Geometry check sheet. Reference: the model listing, model coordinates, mm. A direction names the side the tool comes from. Coordinates: 2 decimals unless noted, no trailing zeros. Write each loop counter-clockwise with the first axis right and the second up, starting at its lowest first coordinate (ties: lowest second). Pieces come first, ordered by that corner, then holes. Notation, with made-up numbers: (19.25, 46.25) -> (47.25, 46.25) arc R5 ccw to (47.25, 54.25) -> close; hole circle Ø7 at (48, -31.75). An arc over 180 degrees is marked (long way). Answer in a Markdown table with one row per item. Add a question column.
Q1. Release check for a two-part mould opening along Z. For faces 1 (the face through (43.909, 4.829, -77.465)), 2 (the face through (-1, 3.683, -1)), 3 (the face through (-45.4, 9.525, -0.4)) record: pulls with the +Z half, pulls with the -Z half, needs draft (parallel to the pull), parting line crosses it, or undercut.
Q2. Gauge pin test, flat ends, axial feed: P1, Ø3, axis at x = -19.5, z = -28, coming from the +Y side; P2, Ø1.4, axis at x = -19.05, y = 1.778, coming from the -Z side; P3, Ø1.8, axis at x = 19.05, y = 1.778, coming from the -Z side. Record the tip position at first contact, or that the pin passes through.
Q3. Thickness scan on line 1 (Y direction, x = -19.05, z = -75.5); line 2 (Z direction, x = 36, y = 4.25) (3 decimals); line 3 (X direction, y = 3.75, z = -24). Record the ranges inside material, lowest first.
Q4. Section check B-B, the plane x = -7. Record the boundary of the cut face in (y, z) (3 decimals), and give its area (3 significant figures).
Q5. Tool access check on faces 4 (the face through (-43.909, 4.829, -77.465)), 5 (the face through (-27.94, 7, -72)), 6 (the face through (-32.447, 7.741, 65.264)). Record the directions out of +Z, -Z, +X, -X, +Y, -Y that give a thin tool (end or side, any length) a straight path to the whole face; none if there is none.
Q6. Section check A-A, the plane z = 62.5. Record the boundary of the cut face in (x, y) (3 decimals), and give its area (3 significant figures).
```python
from build123d import *

# Parameters (mm, degrees)
SKETCH1_W                      = 91.44
SKETCH1_H                      = 158.75
BOSS_EXTRUDE1_DEPTH            = 9.525
FILLET1_R                      = 6.35
SKETCH2_W                      = 86.36
SKETCH2_H                      = 128.524
CUT_EXTRUDE1_DEPTH             = 5.842
F_4_40_TAPPED_HOLE1_AT_2_COUNT = 2
F_4_40_TAPPED_HOLE1_AT_2_PITCH = 38.1
SKETCH7_R                      = 3.175
CUT_EXTRUDE2_DEPTH             = 5.842
CHAMFER1_SIZE                  = 2.032
CHAMFER1_SIZE2                 = 3.519527241
CUT_EXTRUDE3_REACH             = 94.095
SKETCH8_W                      = 55.88
SKETCH8_H                      = 158.75


with BuildPart() as part:
    # Sketch1 → Boss-Extrude1 (new body)
    with BuildSketch(Plane(origin=(0, 0, 0), x_dir=(1, 0, 0), z_dir=(0, 1, 0))):
        Rectangle(SKETCH1_W, SKETCH1_H)
    extrude(amount=BOSS_EXTRUDE1_DEPTH)

    # Fillet1
    fillet1_edges = [part.edges().sort_by_distance(p)[0] for p in [
        (45.72, 4.7625, 79.375),
        (-45.72, 4.7625, 79.375),
        (-45.72, 4.7625, -79.375),
        (45.72, 4.7625, -79.375),
    ]]
    fillet(fillet1_edges, radius=FILLET1_R)

    # Sketch2 → Cut-Extrude1 (cut)
    with BuildSketch(Plane(origin=(0, 9.525, 0), x_dir=(1, 0, 0), z_dir=(0, 1, 0))):
        Rectangle(SKETCH2_W, SKETCH2_H)
    extrude(amount=-CUT_EXTRUDE1_DEPTH, mode=Mode.SUBTRACT)

    # Sketch5 → #4-40 Tapped Hole1 (revolve, cut)
    with BuildSketch(Plane(origin=(-19.05, 1.778, 79.375), x_dir=(0, -1, 0), z_dir=(1, 0, 0))):
        Polygon((0, 0), (0, 8.273752758), (1.1303, 7.5946), (1.1303, 0), align=None)
    f_4_40_tapped_hole1 = revolve(axis=Axis((-19.05, 1.778, 85.725), (0, 0, -1)), mode=Mode.SUBTRACT)

    # #4-40 Tapped Hole1 at 2: #4-40 Tapped Hole1 ×2
    with Locations(*[(i * F_4_40_TAPPED_HOLE1_AT_2_PITCH, 0, 0) for i in range(1, F_4_40_TAPPED_HOLE1_AT_2_COUNT)]):
        add(f_4_40_tapped_hole1, mode=Mode.SUBTRACT)

    # Sketch7 → Cut-Extrude2 (cut)
    with BuildSketch(Plane(origin=(0, 9.525, 0), x_dir=(1, 0, 0), z_dir=(0, 1, 0))):
        with Locations((-40.005, 64.262)):
            Circle(SKETCH7_R)
        with Locations((40.005, 64.262)):
            Circle(SKETCH7_R)
        with Locations((-40.005, -64.262)):
            Circle(SKETCH7_R)
        with Locations((40.005, -64.262)):
            Circle(SKETCH7_R)
    extrude(amount=-CUT_EXTRUDE2_DEPTH, mode=Mode.SUBTRACT)

    # Mirror1: #4-40 Tapped Hole1 across plane
    add(f_4_40_tapped_hole1.mirror(Plane.XY), mode=Mode.SUBTRACT)

    # Mirror1 copy 1 sketch → Mirror1 copy 1 (revolve, cut)
    with BuildSketch(Plane(origin=(19.05, 1.778, -79.375), x_dir=(0, -1, 0), z_dir=(1, 0, 0))):
        Polygon((0, 0), (0, -8.273752758), (1.1303, -7.5946), (1.1303, 0), align=None)
    revolve(axis=Axis((19.05, 1.778, -85.725), (0, 0, -1)), mode=Mode.SUBTRACT)

    # Chamfer1
    chamfer1_edges = [part.edges().sort_by_distance(p)[0] for p in [
        (43.18, 9.525, 0),
        (-43.18, 9.525, 0),
        (0, 9.525, -64.262),
        (0, 9.525, 64.262),
        (40.005, 9.525, -67.437),
        (-40.005, 9.525, 67.437),
        (40.005, 9.525, 67.437),
        (-40.005, 9.525, -67.437),
    ]]
    chamfer1_side = [part.faces().sort_by_distance(p)[0] for p in [
        (0, 9.525, -77.542983731),
    ]]
    chamfer(chamfer1_edges, length=CHAMFER1_SIZE, length2=CHAMFER1_SIZE2, reference=chamfer1_side[0])

    # Cut-Extrude3: up to this face of the body (flat: up to its plane)
    cut_extrude3_end = Plane(part.part.faces().sort_by_distance((0, 3.683, 0))[0])
    # Sketch8 → Cut-Extrude3 (cut, up to the picked face)
    with BuildSketch(Plane(origin=(0, 9.525, 0), x_dir=(1, 0, 0), z_dir=(0, 1, 0)), mode=Mode.PRIVATE) as cut_extrude3_sk1:
        Rectangle(SKETCH8_W, SKETCH8_H)
    cut_extrude3_tool1 = split(extrude(cut_extrude3_sk1.sketch, amount=-CUT_EXTRUDE3_REACH, mode=Mode.PRIVATE), bisect_by=cut_extrude3_end, keep=Keep.BOTH, mode=Mode.PRIVATE)
    add(cut_extrude3_tool1.solids().sort_by(Axis((0, 9.525, 0), (0, -1, 0)))[0], mode=Mode.SUBTRACT)


solid = part.part
```
Calculated:
| question | item | result |
|---|---|---|
| 1 | face 1 | pulls with the -Z half |
| 1 | face 2 | undercut |
| 1 | face 3 | needs draft |
| 2 | P1 | stops at y = 3.68 |
| 2 | P2 | stops at z = -71.52 |
| 2 | P3 | stops at z = -71.64 |
| 3 | line 1 | y = 0 to 0.65, 2.91 to 3.68 |
| 3 | line 2 | z = -79.375 to -64.262, 64.262 to 79.375 |
| 3 | line 3 | x = -45.72 to -43.18, 43.18 to 45.72 |
| 4 | outline | (0, -79.375) -> (3.683, -79.375) -> (3.683, 79.375) -> (0, 79.375) -> close |
| 4 | area | 585 mm² |
| 5 | face 4 | -Z, -X, +Y, -Y |
| 5 | face 5 | +Z, -Z, +Y |
| 5 | face 6 | +Y |
| 6 | outline | (-45.72, 0) -> (45.72, 0) -> (45.72, 9.525) -> (45.212, 9.525) -> (43.18, 6.005) -> (43.18, 3.683) -> (-43.18, 3.683) -> (-43.18, 6.005) -> (-45.212, 9.525) -> (-45.72, 9.525) -> close |
| 6 | area | 359 mm² |
